Autodesk Inventor part; units mm, degrees
ref_plane "YZ Plane" through (0, 0, 0) normal (1, 0, 0) x (0, 1, 0)
ref_plane "XZ Plane" through (0, 0, 0) normal (0, 1, 0) x (-1, 0, 0)
ref_plane "XY Plane" through (0, 0, 0) normal (0, 0, 1) x (1, 0, 0)
sketch "Sketch1" plane through (0, 0, 0) normal (0, 1, 0) x (-1, 0, 0)
  line L0 (-17, -97) -> (17, -97)
  line L1 (17, -97) -> (17, 97)
  line L2 (17, 97) -> (-17, 97)
  line L3 (-17, 97) -> (-17, -97)
  line L4 (-17, -97) -> (17, 97) construction
  line L5 (17, -97) -> (-17, 97) construction
  point P0 (0, 0)
  dimension "d0" = 34
  dimension "d1" = 194
extrude "Extrusion1" add sketch "Sketch1" along normal blind 3
sketch "Sketch2" plane through (0, 0, 0) normal (0, -1, 0) x (1, 0, 0)
  line L0 (14, 94) -> (-14, 94)
  line L1 (-14, 94) -> (-14, -94)
  line L2 (-14, -94) -> (14, -94)
  line L3 (14, -94) -> (14, 94)
  line L4 (14, 94) -> (-14, -94) construction
  line L5 (-14, 94) -> (14, -94) construction
  line L6 (-17, -97) -> (-17, 97)
  line L7 (17, -97) -> (-17, -97)
  point P0 (0, 0)
  dimension "d4" = 3
  dimension "d5" = 3
extrude "Extrusion2" add sketch "Sketch2" along normal blind 3
fillet "Fillet1" radius 2 8 edges at (17, 1.5, 97) (14, -1.5, 94) (-14, -1.5, 94) (-17, 1.5, 97) (14, -1.5, -94) (17, 1.5, -97) (-17, 1.5, -97) (-14, -1.5, -94)
fillet "Fillet2" radius 0.5 8 edges at (-13.4142, -3, 93.4142) (-14, -3, 0) (-13.4142, -3, -93.4142) (0, -3, -94) (13.4142, -3, -93.4142) (14, -3, 0) (13.4142, -3, 93.4142) (0, -3, 94)
properties part number "module-lid_switch"
Geometry: final body of the model. Coordinates: model frame, mm. Round coordinates to 2 decimals unless told otherwise and drop trailing zeros. Order: outer loops, then holes, each group sorted by start corner. A loop starts at its lowest first (then second) coordinate and runs counter-clockwise, first axis right, second up. Notation, with made-up numbers: (20, -26) - (76, -26) arc R25 cw to (76, -6) - close; hole circle Ø2 at (-13.75, 58.5). An arc over 180 degrees is marked (long way). Use CSV: the item, a comma, the result in double quotes. Start each with the question number.
Q1. Mould query, pull axis X, two halves, no side actions, for faces 1 (the face through (-17, 1, -1)), 2 (the face through (17, 1, 1)), 3 (the face through (0, -3, 1)). Classes: +X half, -X half, draft (parallel to the pull), parting line (faces both ways), or undercut.
Q2. First-contact query: pin 1 (0.8 mm diameter, centred on x = -5, y = -2, fed in from -Z). Flat tip, straight axial feed; report the tip coordinate or a pass-through.
Q3. Material intervals for line 1 along X through (y, z) = (-0.5, -59); line 2 along Z through (x, y) = (10, -1.25); line 3 along Z through (x, y) = (-12.5, -2.25), sorted ascending. Write a range as from..to.
Q4. Section query A-A (x = -3). Return loops of the section in (y, z), and give its area (3 significant figures).
Q5. Section query C-C (y = -1.5). Return loops of the section in (x, z).
Q6. Section query B-B (z = 10). Return loops of the section in (x, y).
Result set:
1,face 1,"-X half"
1,face 2,"+X half"
1,face 3,"draft"
2,pin 1,"stops at z = -94"
3,line 1,"x = -14..14"
3,line 2,"z = -94..94"
3,line 3,"z = -93.94..93.94"
4,outline,"(-3, -93.5) arc R0.5 ccw to (-2.5, -94) - (0, -94) - (0, -97) - (3, -97) - (3, 97) - (0, 97) - (0, 94) - (-2.5, 94) arc R0.5 ccw to (-3, 93.5) - close"
4,area,"1,150 mm2"
5,outline,"(-14, -92) arc R2 ccw to (-12, -94) - (12, -94) arc R2 ccw to (14, -92) - (14, 92) arc R2 ccw to (12, 94) - (-12, 94) arc R2 ccw to (-14, 92) - close"
6,outline,"(-17, 0) - (-14, 0) - (-14, -2.5) arc R0.5 ccw to (-13.5, -3) - (13.5, -3) arc R0.5 ccw to (14, -2.5) - (14, 0) - (17, 0) - (17, 3) - (-17, 3) - close"
